The figure shows three views and two pictorial views of one solid part (mm, origin at its lowest corner). Answer the questions. Coordinates: 2 decimals unless noted, no trailing zeros. Write each loop counter-clockwise with the first axis right and the second up, starting at its lowest first coordinate (ties: lowest second). Pieces come first, ordered by that corner, then holes.
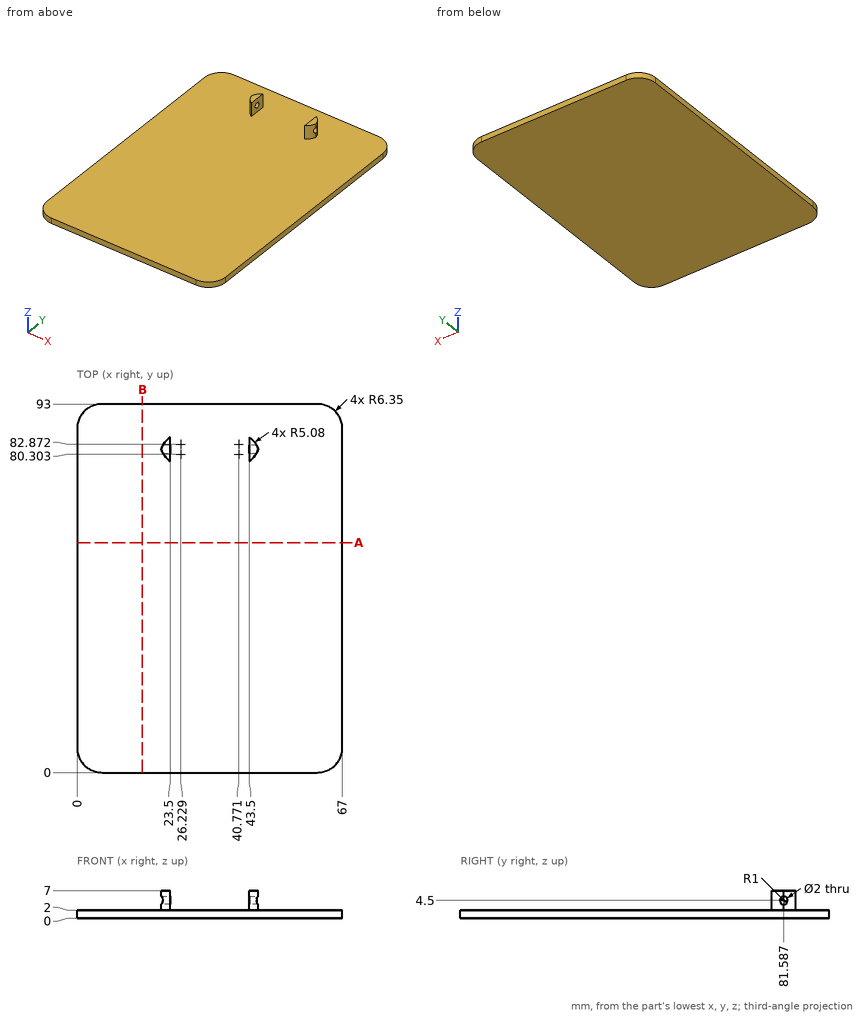
1. Section A-A on y = 58 is taken. Give the vertices of the cut face in (x, z).
Results found:
outline: (0, 0) - (67, 0) - (67, 2) - (0, 2) - close
2. Section B-B on x = 16.5 is taken. Give the vertices of the cut face in (y, z), then the cut area to 3 significant figures.
Results found:
outline: (0, 0) - (93, 0) - (93, 2) - (0, 2) - close
area: 186 mm2
3. Find the intervals of material crossed by L1, parallel to Z at x = 5.5, y = 65.5; L2, parallel to Y at x = 45.2, z = 4.5 (1 decimal); L3, parallel to Y at x = 22.55, z = 4.5 (1 decimal), in increasing order.
Results found:
L1: z = 0 to 2
L2: y = 80.4 to 80.6, 82.6 to 82.8
L3: y = 79.4 to 80.6, 82.6 to 83.8
4. Flat-ended cylindrical pins translate along their axes: P1, Ø1.5, axis at y = 80, z = 4.5, coming from the +X side; P2, Ø2.5, axis at y = 81.59, z = 4.5, coming from the -X side; P3, Ø3, axis at x = 24.5, z = 4, coming from the -Y side. Find the tip coordinate at first contact, or state that the pin passes through.
Results found:
P1: stops at x = 45.34
P2: stops at x = 21.31
P3: stops at y = 78.59
